```python
from build123d import *

# Parameters (mm, degrees)
ESBO_O1_W                = 28
ESBO_O1_H                = 53
RESSALTO_EXTRUS_O1_DEPTH = 0.45
CORTE_EXTRUS_O1_REACH    = 31.984
ESBO_O4_R                = 1.5
CORTE_EXTRUS_O2_REACH    = 31.984
ESBO_O5_R                = 0.5
PADR_O_LINEAR1_COUNT     = 14
PADR_O_LINEAR1_PITCH     = 2.54


with BuildPart() as part:
    # Esbo_o1 → Ressalto-extrus_o1 (new, symmetric)
    with BuildSketch(Plane.XY):
        Rectangle(ESBO_O1_W, ESBO_O1_H)
    extrude(amount=RESSALTO_EXTRUS_O1_DEPTH, both=True)

    # Esbo_o4 → Corte-extrus_o1 (cut, up to next)
    with BuildSketch(Plane.XY.offset(0.45), mode=Mode.PRIVATE) as corte_extrus_o1_sk1:
        with Locations((-11.5, -24)):
            Circle(ESBO_O4_R)
    corte_extrus_o1_tool1 = extrude(corte_extrus_o1_sk1.sketch, amount=-CORTE_EXTRUS_O1_REACH, mode=Mode.PRIVATE) & part.part
    # Esbo_o4 → Corte-extrus_o1 (cut, up to next)
    with BuildSketch(Plane.XY.offset(0.45), mode=Mode.PRIVATE) as corte_extrus_o1_sk2:
        with Locations((11.5, -24)):
            Circle(ESBO_O4_R)
    corte_extrus_o1_tool2 = extrude(corte_extrus_o1_sk2.sketch, amount=-CORTE_EXTRUS_O1_REACH, mode=Mode.PRIVATE) & part.part
    # Esbo_o4 → Corte-extrus_o1 (cut, up to next)
    with BuildSketch(Plane.XY.offset(0.45), mode=Mode.PRIVATE) as corte_extrus_o1_sk3:
        with Locations((11.5, 24)):
            Circle(ESBO_O4_R)
    corte_extrus_o1_tool3 = extrude(corte_extrus_o1_sk3.sketch, amount=-CORTE_EXTRUS_O1_REACH, mode=Mode.PRIVATE) & part.part
    # Esbo_o4 → Corte-extrus_o1 (cut, up to next)
    with BuildSketch(Plane.XY.offset(0.45), mode=Mode.PRIVATE) as corte_extrus_o1_sk4:
        with Locations((-11.5, 24)):
            Circle(ESBO_O4_R)
    corte_extrus_o1_tool4 = extrude(corte_extrus_o1_sk4.sketch, amount=-CORTE_EXTRUS_O1_REACH, mode=Mode.PRIVATE) & part.part
    add(corte_extrus_o1_tool1.solids().sort_by_distance((-11.5, -24, 0.45))[0], mode=Mode.SUBTRACT)
    add(corte_extrus_o1_tool2.solids().sort_by_distance((11.5, -24, 0.45))[0], mode=Mode.SUBTRACT)
    add(corte_extrus_o1_tool3.solids().sort_by_distance((11.5, 24, 0.45))[0], mode=Mode.SUBTRACT)
    add(corte_extrus_o1_tool4.solids().sort_by_distance((-11.5, 24, 0.45))[0], mode=Mode.SUBTRACT)

    # Esbo_o5 → Corte-extrus_o2 (cut, up to next)
    with BuildSketch(Plane.XY.offset(0.45), mode=Mode.PRIVATE) as corte_extrus_o2_sk1:
        with Locations((-11.5, -21)):
            Circle(ESBO_O5_R)
    corte_extrus_o2_tool1 = extrude(corte_extrus_o2_sk1.sketch, amount=-CORTE_EXTRUS_O2_REACH, mode=Mode.PRIVATE) & part.part
    # Esbo_o5 → Corte-extrus_o2 (cut, up to next)
    with BuildSketch(Plane.XY.offset(0.45), mode=Mode.PRIVATE) as corte_extrus_o2_sk2:
        with Locations((11.5, -21)):
            Circle(ESBO_O5_R)
    corte_extrus_o2_tool2 = extrude(corte_extrus_o2_sk2.sketch, amount=-CORTE_EXTRUS_O2_REACH, mode=Mode.PRIVATE) & part.part
    corte_extrus_o2_1 = corte_extrus_o2_tool1.solids().sort_by_distance((-11.5, -21, 0.45))[0]
    add(corte_extrus_o2_1, mode=Mode.SUBTRACT)
    corte_extrus_o2_2 = corte_extrus_o2_tool2.solids().sort_by_distance((11.5, -21, 0.45))[0]
    add(corte_extrus_o2_2, mode=Mode.SUBTRACT)
    corte_extrus_o2 = corte_extrus_o2_1 + corte_extrus_o2_2  # Corte-extrus_o2 as one shape, for the pattern or mirror that repeats it

    # Padr_o linear1: Corte-extrus_o2 ×14
    with Locations(*[(0, i * PADR_O_LINEAR1_PITCH, 0) for i in range(1, PADR_O_LINEAR1_COUNT)]):
        add(corte_extrus_o2, mode=Mode.SUBTRACT)


solid = part.part
```
Design review of the part built by this model. Coordinates are the model's own, in mm. Coordinates: 2 decimals unless noted, no trailing zeros. Write each loop counter-clockwise with the first axis right and the second up, starting at its lowest first coordinate (ties: lowest second). Pieces come first, ordered by that corner, then holes.
1) Mouldability with a two-part tool opening along X and no side actions: class faces 1 (the flat face through (-14, 0, 0)), 2 (the cylindrical face through (11, -21, 0)), 3 (the flat face through (0, 0, -0.45)) as +X half, -X half, draft (parallel to the pull), parting line (faces both ways), or undercut.
2) To check wall thickness, follow L1, parallel to X at y = -10.5, z = 0.2; L2, parallel to Y at x = -10.5, z = -0.1; L3, parallel to Y at x = 10.25, z = 0. State the ranges of each line that lie inside material, in increasing order.
3) Add section A-A (y = 24). Write out the cut boundary in (x, z).
4) Add section C-C (y = -13.38). Write out the cut boundary in (x, z), plus the area to 3 significant figures.
5) Insertion check: pin 1 (4 mm diameter, centred on x = 11.5, y = 24, fed in from -Z). The pin has a flat end and moves straight along its axis. Give the tip position at first contact, or say it passes through.
6) Add section B-B (x = 11.5). State how many separate pieces and enclosed holes the cut face has, plus the area to 3 significant figures.
Check result:
1. face 1: -X half
1. face 2: undercut
1. face 3: draft
2. L1: x = -14 to -11.87, -11.13 to 11.13, 11.87 to 14
2. L2: y = -26.5 to -25.12, -22.88 to 22.88, 25.12 to 26.5
2. L3: y = -26.5 to -24.83, -23.17 to 23.17, 24.83 to 26.5
3. outline: (-14, -0.45) - (-13, -0.45) - (-13, 0.45) - (-14, 0.45) - close; (-10, -0.45) - (10, -0.45) - (10, 0.45) - (-10, 0.45) - close; (13, -0.45) - (14, -0.45) - (14, 0.45) - (13, 0.45) - close
4. outline: (-14, -0.45) - (-12, -0.45) - (-12, 0.45) - (-14, 0.45) - close; (-11, -0.45) - (11, -0.45) - (11, 0.45) - (-11, 0.45) - close; (12, -0.45) - (14, -0.45) - (14, 0.45) - (12, 0.45) - close
4. area: 23.4 mm2
5. pin 1: stops at z = -0.45
6. separate pieces: 17
6. enclosed holes: 0
6. area: 29.7 mm2
